For this review, take the finished solid that the model builds, in its own axes (mm). A direction names the side the tool comes from. Coordinates: 2 decimals unless noted, no trailing zeros. Loops run counter-clockwise (first coordinate to the right, second up) from the corner with the lowest first, then second, coordinate; pieces in that order, holes last.
1. Take a section at A-A, the plane y = 0. State the section outline as (x, z) points, then the cut area to 3 significant figures.
2. To check wall thickness, follow probe 1 along Y at (x, z) = (-16.5, 50.7); probe 2 along Z at (x, y) = (-16, 4); probe 3 along Y at (x, z) = (-14.75, 51.4). State the ranges of each line that lie inside material, in increasing order.
3. Mouldability with a two-part tool opening along X and no side actions: class faces 1 (the face through (-13.68, 0.07, 51.67)), 2 (the face through (-17, 0, 53.242)), 3 (the face through (-11.18, -0.18, 51.41)) as pulls with the +X half, pulls with the -X half, needs draft (parallel to the pull), parting line crosses it, or undercut.
4. Take a section at C-C, the plane z = 52.75. State the section outline as (x, y) points, then the cut area to 3 significant figures.
5. Clearance check with a flat-ended pin moving along its axis: P1, Ø2, axis at x = -14, y = 0.5, coming from the -Z side. State where the tip first meets the part, or that it passes through.
6. Take a section at B-B, the plane x = -16. State the section outline as (y, z) points.
7. Machinability: for faces 4 (the face through (-14, 4, 52.642)), 5 (the face through (-17, 0, 50.137)), which of the approach directions +Z, -Z, +X, -X, +Y, -Y give a long, thin tool a straight path to every point of the face, cutting with its end or side? Answer none if there is none.
8. Take a section at D-D, the plane x = -12.25. State the section outline as (y, z) points.
Autodesk Inventor part; units mm, degrees
ref_plane "YZ Plane" through (0, 0, 0) normal (1, 0, 0) x (0, 1, 0)
ref_plane "XZ Plane" through (0, 0, 0) normal (0, 1, 0) x (-1, 0, 0)
ref_plane "XY Plane" through (0, 0, 0) normal (0, 0, 1) x (1, 0, 0)
sketch "Sketch1" plane through (0, 0, 0) normal (0, 1, 0) x (-1, 0, 0)
  line L0 (16.6772, 52.6366) -> (16.6772, 50.1366)
  line L1 (16.6772, 50.1366) -> (19.1772, 50.1366)
  line L2 (19.1772, 50.1366) -> (19.1772, 52.6421)
  line L3 (19.1772, 52.6421) -> (19.7772, 52.6421)
  line L4 (19.7772, 52.6421) -> (19.7772, 53.2421)
  line L5 (19.7772, 53.2421) -> (16.6772, 53.2421)
  line L6 (16.6772, 53.2421) -> (16.6772, 52.6366)
  line L7 (15.1772, 53.2421) -> (15.1772, 48.9703)
  point P0 (0, 0)
  dimension "d0" = 2.5
  dimension "d1" = 1.5
  dimension "d2" = 2.5
  dimension "d3" = 0.6
  dimension "d4" = 0.6
  dimension "d5" = 0
revolve "Revolution1" add sketch "Sketch1" angle 360 about axis through (-15.1772, 0, 53.2421) along (0, 0, -1)
properties part number "00_ballbearing_8mm"
Results list:
1. outline: (-19.78, 52.64) - (-19.18, 52.64) - (-19.18, 50.14) - (-16.68, 50.14) - (-16.68, 53.24) - (-19.78, 53.24) - close; (-13.68, 50.14) - (-11.18, 50.14) - (-11.18, 52.64) - (-10.58, 52.64) - (-10.58, 53.24) - (-13.68, 53.24) - close
1. area: 16.2 mm2
2. probe 1: y = -3.77 to -0.71, 0.71 to 3.77
2. probe 2: z = 52.64 to 53.24
2. probe 3: y = -3.98 to -1.44, 1.44 to 3.98
3. face 1: undercut
3. face 2: needs draft
3. face 3: parting line crosses it
4. outline: circle Ø9.2 at (-15.18, 0); hole circle Ø3 at (-15.18, 0)
4. area: 59.4 mm2
5. P1: stops at z = 50.14
6. outline: (-4.53, 52.64) - (-3.91, 52.64) - (-3.91, 50.14) - (-1.25, 50.14) - (-1.25, 53.24) - (-4.53, 53.24) - close; (1.25, 50.14) - (3.91, 50.14) - (3.91, 52.64) - (4.53, 52.64) - (4.53, 53.24) - (1.25, 53.24) - close
7. face 4: -Z
7. face 5: -Z, +X, -X, +Y, -Y
8. outline: (-3.55, 52.64) - (-2.73, 52.64) - (-2.73, 50.14) - (2.73, 50.14) - (2.73, 52.64) - (3.55, 52.64) - (3.55, 53.24) - (-3.55, 53.24) - close
